from build123d import *

# Parameters (mm, degrees)
EXTRUDE1_DEPTH                 = 8
EXTRUDE2_DEPTH                 = 8
SKETCH4_W                      = 6
SKETCH4_H                      = 60
EXTRUDE3_DEPTH                 = 10
F_4_0_4_DIAMETER_HOLE2_D       = 4
F_4_0_4_DIAMETER_HOLE2_DEPTH   = 15
SKETCH6_W                      = 9
SKETCH6_H                      = 30
EXTRUDE4_DEPTH                 = 12
F_5_0_5_DIAMETER_HOLE1_D       = 5
F_2_9_2_9_DIAMETER_HOLE1_D     = 2.9
F_2_9_2_9_DIAMETER_HOLE1_DEPTH = 10
SKETCH10_R                     = 12.5
EXTRUDE5_DEPTH                 = 10
F_2_9_2_9_DIAMETER_HOLE2_D     = 2.9
F_2_9_2_9_DIAMETER_HOLE2_DEPTH = 10
EXTRUDE8_DEPTH                 = 21
SKETCH15_W                     = 60
SKETCH15_H                     = 25
EXTRUDE9_DEPTH                 = 4
F_4_0_4_DIAMETER_HOLE4_D       = 3.9
F_4_0_4_DIAMETER_HOLE4_DEPTH   = 15
F_4_0_4_DIAMETER_HOLE5_D       = 3.9
F_4_0_4_DIAMETER_HOLE5_DEPTH   = 15


with BuildPart() as part:
    # Sketch1 → Extrude1 (new body)
    with BuildSketch(Plane.XY):
        Polygon((-40, -10), (-25, 40), (25, 40), (40, -10), (90, -10), (90, -40), (-90, -40), (-90, -10), align=None)
    extrude(amount=EXTRUDE1_DEPTH)

    # Sketch2 → Extrude2 (add)
    with BuildSketch(Plane.XY):
        Polygon((-50, -40), (50, -40), (30, -73.244533262), (30, -80), (-30, -80), (-30, -73.244533262), align=None)
    extrude(amount=EXTRUDE2_DEPTH)

    # Sketch4 → Extrude3 (add)
    with BuildSketch(Plane.XY.offset(8)):
        with Locations((0, -10)):
            Rectangle(SKETCH4_W, SKETCH4_H)
    extrude(amount=EXTRUDE3_DEPTH)

    # Ø4.0 (4) Diameter Hole2
    with Locations(Plane(origin=(25, -3, 0), x_dir=(-1, 0, 0), z_dir=(0, 0, -1))):
        with Locations((0, 0), (50, 0), (0, 20), (50, 20)):
            Hole(F_4_0_4_DIAMETER_HOLE2_D / 2, depth=F_4_0_4_DIAMETER_HOLE2_DEPTH)

    # Sketch6 → Extrude4 (add)
    with BuildSketch(Plane.XY.offset(8)):
        with Locations((-85.5, -25)):
            Rectangle(SKETCH6_W, SKETCH6_H)
    extrude4 = extrude(amount=EXTRUDE4_DEPTH)

    # Ø5.0 (5) Diameter Hole1 (through all)
    with Locations(Plane(origin=(-85.5, -10, 16), x_dir=(0, 0, 1), z_dir=(0, 1, 0))):
        with Locations((0, 0)):
            f_5_0_5_diameter_hole1 = Hole(F_5_0_5_DIAMETER_HOLE1_D / 2)

    # Mirror1: Extrude4, Ø5.0 (5) Diameter Hole1 across plane
    add(extrude4.mirror(Plane(origin=(0, 0, 0), x_dir=(0, 0, 1), z_dir=(1, 0, 0))))
    add(f_5_0_5_diameter_hole1.mirror(Plane(origin=(0, 0, 0), x_dir=(0, 0, 1), z_dir=(1, 0, 0))), mode=Mode.SUBTRACT)

    # Ø2.9 (2.9) Diameter Hole1
    with Locations(Plane(origin=(-7.5, 40, 4), x_dir=(1, 0, 0), z_dir=(0, 1, 0))):
        with Locations((0, 0), (15, 0)):
            Hole(F_2_9_2_9_DIAMETER_HOLE1_D / 2, depth=F_2_9_2_9_DIAMETER_HOLE1_DEPTH)

    # Sketch10 → Extrude5 (cut)
    with BuildSketch(Plane.XY.offset(8)):
        with Locations((-22.248705181, -27.888411791)):
            Circle(SKETCH10_R)
    extrude5 = extrude(amount=-EXTRUDE5_DEPTH, mode=Mode.SUBTRACT)

    # Mirror2: Extrude5 across plane
    add(extrude5.mirror(Plane(origin=(0, 0, 0), x_dir=(0, 0, 1), z_dir=(1, 0, 0))), mode=Mode.SUBTRACT)

    # Ø2.9 (2.9) Diameter Hole2
    with Locations(Plane(origin=(-3, 12, 13), x_dir=(0, -1, 0), z_dir=(-1, 0, 0))):
        with Locations((0, 0), (44, 0)):
            Hole(F_2_9_2_9_DIAMETER_HOLE2_D / 2, depth=F_2_9_2_9_DIAMETER_HOLE2_DEPTH)

    # Sketch14 → Extrude8 (cut, through all)
    with BuildSketch(Plane(origin=(0, 0, 0), x_dir=(-1, 0, 0), z_dir=(0, 0, -1))):
        Polygon((-30.4, 22), (-15, 22), (-15, 40), (-25, 40), align=None)
        Polygon((25, 40), (15, 40), (15, 22), (30.4, 22), align=None)
    extrude(amount=-EXTRUDE8_DEPTH, mode=Mode.SUBTRACT)

    # Sketch15 → Extrude9 (cut)
    with BuildSketch(Plane.XY.offset(8)):
        with Locations((0, -67.5)):
            Rectangle(SKETCH15_W, SKETCH15_H)
    extrude(amount=-EXTRUDE9_DEPTH, mode=Mode.SUBTRACT)

    # Ø4.0 (4) Diameter Hole4
    with Locations(Plane(origin=(15, -59, 4), x_dir=(1, 0, 0), z_dir=(0, 0, 1))):
        with Locations((0, 0), (-10, -16), (10, -16), (-20, -16), (-40, -16), (-30, 0)):
            Hole(F_4_0_4_DIAMETER_HOLE4_D / 2, depth=F_4_0_4_DIAMETER_HOLE4_DEPTH)

    # Ø4.0 (4) Diameter Hole5
    with Locations(Plane(origin=(0, -48, 8), x_dir=(1, 0, 0), z_dir=(0, 0, 1))):
        with Locations((0, 0)):
            Hole(F_4_0_4_DIAMETER_HOLE5_D / 2, depth=F_4_0_4_DIAMETER_HOLE5_DEPTH)


solid = part.part
Verification items for the finished model (mm, model axes). A direction names the side the tool comes from. Give positions to 0.01 mm unless a question says otherwise; leave off trailing zeros. Write each loop counter-clockwise with the first axis right and the second up, starting at its lowest first coordinate (ties: lowest second). Pieces come first, ordered by that corner, then holes.
(1) Cross-section at B-B (y = -3). Enter the section's corners in (x, z).
(2) Gauge pin test, flat ends, axial feed: pin 1 (3 mm diameter, centred on x = 0, y = -48, fed in from -Z); pin 2 (6 mm diameter, centred on x = -85.5, z = 16, fed in from +Y); pin 3 (3 mm diameter, centred on x = -1.5, z = 14, fed in from +Y); pin 4 (5 mm diameter, centred on x = -15, y = -59, fed in from +Z). Record the tip position at first contact, or that the pin passes through.
(3) Cross-section at D-D (x = 60). Enter the section's corners in (y, z).
(4) Mould release check, pull along X, two halves, no side actions. Record for faces 6 (the face through (-35.267, 5.776, 3.944)), 7 (the face through (15, 31, 4)), 8 (the face through (84, -25, 18)), 9 (the face through (0, 20, 13)): +X half, -X half, draft (parallel to the pull), parting line (faces both ways), or undercut.
(5) Access from +Z, -Z, +X, -X, +Y, -Y to the whole of each face (thin tool, end or side, straight path). Record for faces 1 (the face through (0, -40, 13)), 2 (the face through (0.423, -49.904, 3.944)), 3 (the face through (-71, -10, 5)), 4 (the face through (3, -10, 13)), 5 (the face through (1, -19, 0)).
(6) Material ranges on line 1 (X direction, y = 33, z = 4); line 2 (X direction, y = -32.75, z = 16); line 3 (Z direction, x = 0.05, y = 12), recorded low to high.
(7) Cross-section at A-A (x = -85.5). Enter the section's corners in (y, z), plus the area to 3 significant figures.
(8) Cross-section at C-C (y = -48). Enter the section's corners in (x, z), plus the area to 3 significant figures.
Worked out:
1. outline: (-37.9, 0) - (-27, 0) - (-27, 8) - (-37.9, 8) - close; (-23, 0) - (23, 0) - (23, 8) - (3, 8) - (3, 18) - (-3, 18) - (-3, 8) - (-23, 8) - close; (27, 0) - (37.9, 0) - (37.9, 8) - (27, 8) - close
2. pin 1: passes through
2. pin 2: stops at y = -10
2. pin 3: stops at y = 20
2. pin 4: stops at z = 4
3. outline: (-40, 0) - (-10, 0) - (-10, 8) - (-40, 8) - close
4. face 6: -X half
4. face 7: +X half
4. face 8: undercut
4. face 9: draft
5. face 1: +Z, +X, -X, -Y
5. face 2: +Z, -Z
5. face 3: +Z, -Z, -X, +Y
5. face 4: +Z, +Y, -Y
5. face 5: -Z, +X, -X, +Y, -Y
6. line 1: x = -15 to -8.95, -6.05 to 6.05, 8.95 to 15
6. line 2: x = -90 to -88, -83 to -81, -3 to 3, 81 to 83, 88 to 90
6. line 3: z = 0 to 11.55, 14.45 to 18
7. outline: (-40, 0) - (-10, 0) - (-10, 13.5) - (-40, 13.5) - close; (-40, 18.5) - (-10, 18.5) - (-10, 20) - (-40, 20) - close
7. area: 450 mm2
8. outline: (-45.19, 0) - (-1.95, 0) - (-1.95, 8) - (-45.19, 8) - close; (1.95, 0) - (45.19, 0) - (45.19, 8) - (1.95, 8) - close
8. area: 692 mm2
